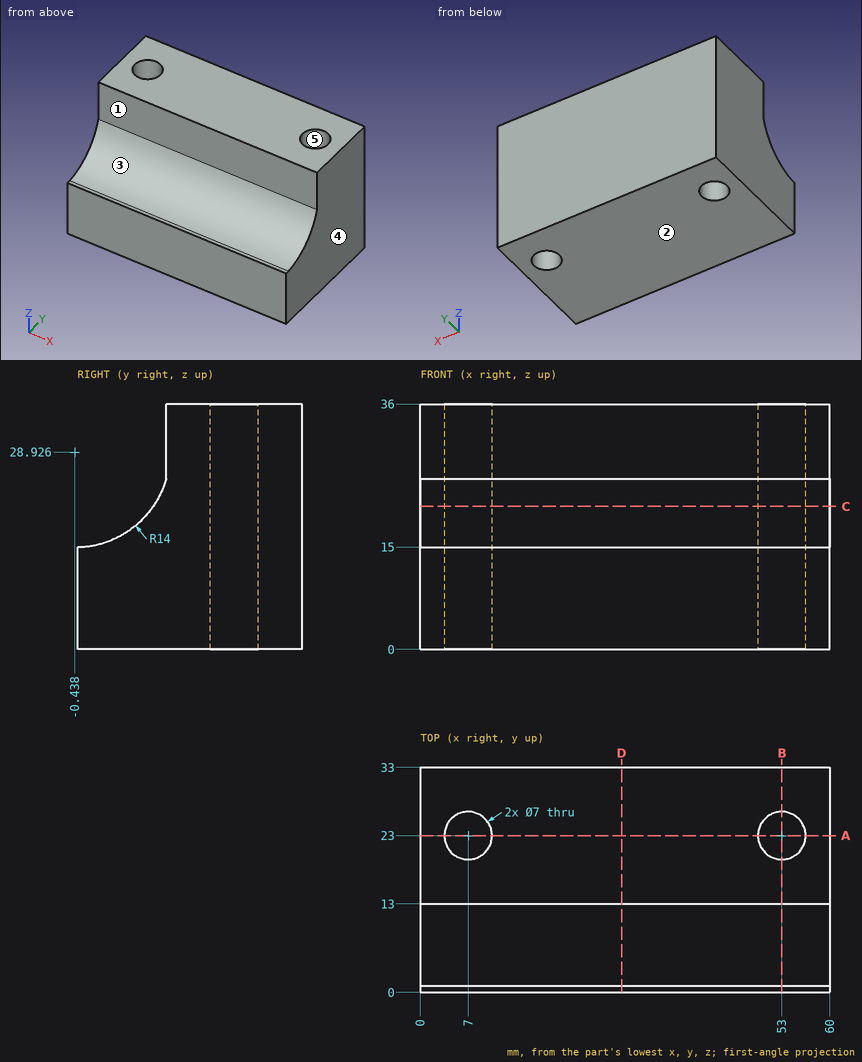
Here's the drawing with two shaded views (mm, measured from the low corner). I have some questions. A direction names the side the tool comes from. Round coordinates to 2 decimals unless told otherwise and drop trailing zeros. Write each loop counter-clockwise with the first axis right and the second up, starting at its lowest first coordinate (ties: lowest second). Pieces come first, ordered by that corner, then holes. Notation, with made-up numbers: M 51,-27 L 73,-27 A19 cw 73,-11 Z; hole C 8.5,51.25 d1. An arc over 180 degrees is marked long. Answer in a Markdown table with one row per item. Add a question column.
Q1. If we mould it in two halves opening along X, with no side actions, what happens to the marked faces 3, 4 and 5? For each: +X half, -X half, draft (parallel to the pull), parting line (faces both ways), or undercut.
Q2. Imagine slicing it at B-B (x = 53). Please give me the cut outline in (y, z), then the cut area to 3 significant figures.
Q3. Imagine slicing it at C-C (z = 21). Please give me the cut outline in (x, y).
Q4. Imagine slicing it at A-A (y = 23). Please give me the cut outline in (x, z), then the cut area to 3 significant figures.
Q5. If I drill on line 1 (X direction, y = 23, z = 9.5); line 2 (Y direction, x = 7, z = 9); line 3 (X direction, y = 22, z = 18.5), over which ranges is the centre line in solid material (lowest first)? Write a range as from..to.
Q6. Imagine slicing it at D-D (x = 29.5). Please give me the cut outline in (y, z), then the cut area to 3 significant figures.
Q7. On a 3-axis mill with a long thin cutter (end or side, diameter ignored), from which of +Z, -Z, +X, -X, +Y, -Y can I reach the whole of each face in a straight line? I mean the marked faces 1 and 2. Say none if no direction works.
Q8. Will these pins go through, and if not, where does the flat tip stop? pin 1 Ø1.5 at (x, z) = (35.5, 29) entering from -Y; pin 2 Ø5.5 at (x, y) = (53, 23) entering from -Z.
Values:
| question | item | result |
|---|---|---|
| 1 | face 3 | draft |
| 1 | face 4 | +X half |
| 1 | face 5 | undercut |
| 2 | outline | M 0,0 L 19.5,0 L 19.5,36 L 13,36 L 13,25 A14 cw 1,15 L 0,15 Z; M 26.5,0 L 33,0 L 33,36 L 26.5,36 Z |
| 2 | area | 698 mm^2 |
| 3 | outline | M 0,11.1 L 60,11.1 L 60,33 L 0,33 Z; hole C 7,23 d7; hole C 53,23 d7 |
| 4 | outline | M 0,0 L 3.5,0 L 3.5,36 L 0,36 Z; M 10.5,0 L 49.5,0 L 49.5,36 L 10.5,36 Z; M 56.5,0 L 60,0 L 60,36 L 56.5,36 Z |
| 4 | area | 1,660 mm^2 |
| 5 | line 1 | 0..3.5, 10.5..49.5, 56.5..60 |
| 5 | line 2 | 0..19.5, 26.5..33 |
| 5 | line 3 | 0..3.65, 10.35..49.65, 56.35..60 |
| 6 | outline | M 0,0 L 33,0 L 33,36 L 13,36 L 13,25 A14 cw 1,15 L 0,15 Z |
| 6 | area | 950 mm^2 |
| 7 | face 1 | +Z, +X, -X, -Y |
| 7 | face 2 | -Z, +X, -X, +Y, -Y |
| 8 | pin 1 | y = 13 |
| 8 | pin 2 | through |
